For this review, use the dimensioned drawing (mm, ordinates from the lowest corner) and the shaded views. Round coordinates to 2 decimals unless told otherwise and drop trailing zeros. Write each loop counter-clockwise with the first axis right and the second up, starting at its lowest first coordinate (ties: lowest second). Pieces come first, ordered by that corner, then holes. Notation, with made-up numbers: M 83,73.25 L 109,73.25 A18 ccw 109,98.25 Z; hole C 52,7.25 d1. An arc over 180 degrees is marked long. Use one line per item in the form item = value. Start each with the question number.
Item 1: Add section B-B (x = 92.5). State the section outline as (y, z) points.
Item 2: Add section C-C (z = 2.5). Count the separate pieces of the cut face and the enclosed holes in it, and give its area (3 significant figures).
Item 3: Add section D-D (y = 64.5). State the section outline as (x, z) points.
Item 4: For line 1 (Y direction, x = 62, z = 4.15); line 2 (X direction, y = 153, z = 4.75); line 3 (X direction, y = 118.5, z = 3.9), list the stretches that pass through material, from the lowest coordinate up. Write a range as [from, to].
Item 5: Add section A-A (y = 134). State the section outline as (x, z) points.
Item 6: For P1, Ø1, axis at y = 101, z = 3.5, coming from the +X side; P2, Ø2, axis at x = 112, z = 3, coming from the -Y side; P3, Ø1.5, axis at x = 63, z = 1.5, coming from the +Y side, all flat-tipped, find the tip position at first contact; note any pin that passes through.
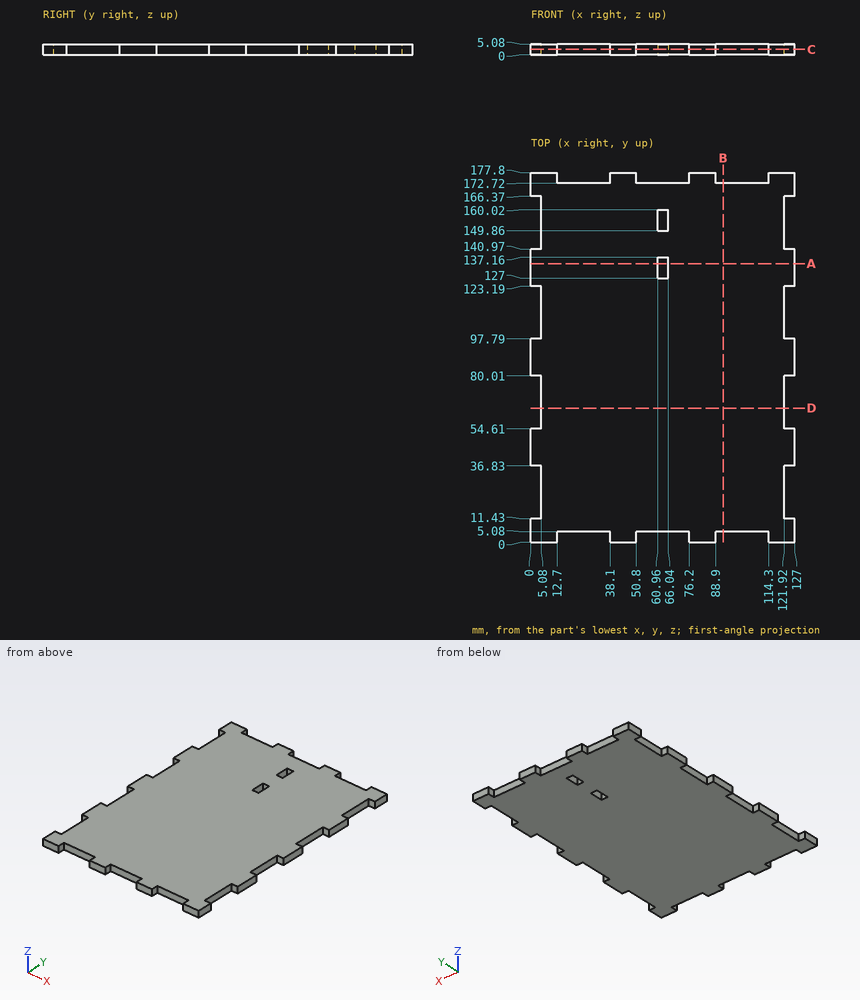
Calculated:
q1.outline = M 5.08,0 L 172.72,0 L 172.72,5.08 L 5.08,5.08 Z
q2.separate_pieces = 1
q2.enclosed_holes = 2
q2.area = 20,700 mm^2
q3.outline = M 5.08,0 L 121.92,0 L 121.92,5.08 L 5.08,5.08 Z
q4.line_1 = [5.08, 127], [137.16, 149.86], [160.02, 172.72]
q4.line_2 = [5.08, 60.96], [66.04, 121.92]
q4.line_3 = [5.08, 121.92]
q5.outline = M 0,0 L 60.96,0 L 60.96,5.08 L 0,5.08 Z; M 66.04,0 L 127,0 L 127,5.08 L 66.04,5.08 Z
q6.P1 = 121.92
q6.P2 = 5.08
q6.P3 = 172.72
